```python
from build123d import *

# Parameters (mm, degrees)
EXTRUDE_3_DEPTH = 17
EXTRUDE_4_DEPTH = 11


with BuildPart() as part:
    # 草圖3 → 填料-伸長3 (new body)
    with BuildSketch(Plane.XY):
        Polygon((0, 0), (64, 0), (64, 18.861561237), (40, 32.717967697), (0, 22), align=None)
    extrude(amount=-EXTRUDE_3_DEPTH)

    # 草圖4 → 填料-伸長4 (add)
    with BuildSketch(Plane.XY):
        Polygon((0, 0), (32, 0), (32, 13.425625842), (0, 22), align=None)
    extrude(amount=EXTRUDE_4_DEPTH)


solid = part.part
```
Geometry check sheet. Reference: the model listing, model coordinates, mm. A direction names the side the tool comes from. Coordinates: 2 decimals unless noted, no trailing zeros. Write each loop counter-clockwise with the first axis right and the second up, starting at its lowest first coordinate (ties: lowest second). Pieces come first, ordered by that corner, then holes. Notation, with made-up numbers: M -18,-17 L 6,-17 A10 ccw 6,-7 Z; hole C 17,30 d5. An arc over 180 degrees is marked long. Use one line per item in the form item = value. Start each with the question number.
1) Go/stop test with a flat-tipped pin: pin 1 Ø2 at (y, z) = (21.5, -1) entering from +X. Record where the tip stops, or that it passes through.
2) Section check A-A on z = 4. Enter the section's corners in (x, y), and give its area (3 significant figures).
3) Section check B-B on x = 5.5. Enter the section's corners in (y, z).
4) Thickness scan on probe 1 along Z at (x, y) = (36.5, 30); probe 2 along X at (y, z) = (8, 0.5); probe 3 along Y at (x, z) = (17, -7). Record the ranges inside material, lowest first. Write a range as from..to.
5) Section check C-C on y = 6. Enter the section's corners in (x, z), and give its area (3 significant figures).
6) Set-up check for faces 1 (the flat face through (39, 17, 0)), 2 (the flat face through (32, 7, 5)), 3 (the flat face through (32, 13, -17)): record each of +Z, -Z, +X, -X, +Y, -Y from which the full face is reachable in a straight line by a thin tool's end or side.
7) Section check D-D on z = -3.5. Enter the section's corners in (x, y).
Responses:
q1.pin_1 = 61.16
q2.outline = M 0,0 L 32,0 L 32,13.43 L 0,22 Z
q2.area = 567 mm2
q3.outline = M 0,-17 L 23.47,-17 L 23.47,0 L 20.53,0 L 20.53,11 L 0,11 Z
q4.probe_1 = -17..0
q4.probe_2 = 0..32
q4.probe_3 = 0..26.56
q5.outline = M 0,-17 L 64,-17 L 64,0 L 32,0 L 32,11 L 0,11 Z
q5.area = 1,440 mm2
q6.face_1 = +Z, +X, +Y
q6.face_2 = +Z, +X, +Y, -Y
q6.face_3 = -Z, +X, -X, +Y, -Y
q7.outline = M 0,0 L 64,0 L 64,18.86 L 40,32.72 L 0,22 Z
